Geometry: final body of the model. Coordinates: model frame, mm. Face numbers are marked on the shaded views. A direction names the side the tool comes from. Coordinates: 2 decimals unless noted, no trailing zeros. Order: outer loops, then holes, each group sorted by start corner. A loop starts at its lowest first (then second) coordinate and runs counter-clockwise, first axis right, second up. Notation, with made-up numbers: (-30, 38.25) - (-16, 38.25) arc R24 ccw to (-16, 68.25) - close; hole circle Ø9 at (5, -36.5). An arc over 180 degrees is marked (long way). Use a Markdown table: item, result. Add a question column.
```python
from build123d import *

# Parameters (mm, degrees)
REVOLUCI_N1_ANGLE           = 180
SALIENTE_EXTRUIR1_DEPTH     = 15
CROQUIS4_R                  = 4
CORTAR_EXTRUIR1_DEPTH       = 139.387389496
REVOLUCI_N2_ANGLE           = 10
REVOLUCI_N2_OTHER_WAY_ANGLE = 10
CORTAR_EXTRUIR2_DEPTH       = 10
CROQUIS7_R                  = 2
CORTAR_EXTRUIR3_DEPTH       = 125.891504895
CORTAR_EXTRUIR4_DEPTH       = 141.925841064
REDONDEO1_R                 = 4


with BuildPart() as part:
    # Croquis1 → Revolución1 (revolve)
    with BuildSketch(Plane(origin=(0, 0, 0), x_dir=(0, 0, -1), z_dir=(1, 0, 0))):
        with BuildLine():
            Line((-25.795554958, 35.816642159), (-40.313941934, 90))
            Line((-40.313941934, 90), (-34.102284852, 90))
            Line((-34.102284852, 90), (-20, 37.36955643))
            ThreePointArc((-20, 37.36955643), (-12.468451731, 20.723921943), (0, 7.36955643))
            Line((0, 7.36955643), (0, 0))
            ThreePointArc((0, 0), (-16.178409273, 15.545572574), (-25.795554958, 35.816642159))
        make_face()
    revolve(axis=Axis((0, 7.36955643, 0), (0, -1, 0)), revolution_arc=REVOLUCI_N1_ANGLE)

    # Croquis3 → Saliente-Extruir1 (add)
    with BuildSketch(Plane(origin=(0, 90, 0), x_dir=(1, 0, 0), z_dir=(0, 1, 0))):
        with BuildLine():
            Line((-10, -32.603156782), (-10, -39.053987175))
            ThreePointArc((-10, -39.053987175), (-5.039530881, -39.997712969), (0, -40.313941934))
            Line((0, -40.313941934), (10, -40.313941934))
            Line((10, -40.313941934), (10, -34.102284852))
            Line((10, -34.102284852), (0, -34.102284852))
            ThreePointArc((0, -34.102284852), (-5.055872451, -33.72542047), (-10, -32.603156782))
        make_face()
        with BuildLine():
            Line((-10, 32.603156782), (-10, 39.053987175))
            ThreePointArc((-10, 39.053987175), (-5.039530881, 39.997712969), (0, 40.313941934))
            Line((0, 40.313941934), (10, 40.313941934))
            Line((10, 40.313941934), (10, 34.102284852))
            Line((10, 34.102284852), (0, 34.102284852))
            ThreePointArc((0, 34.102284852), (-5.055872451, 33.72542047), (-10, 32.603156782))
        make_face()
    extrude(amount=SALIENTE_EXTRUIR1_DEPTH)

    # Croquis4 → Cortar-Extruir1 (cut, through all)
    with BuildSketch(Plane.XY.offset(40.313941934)):
        with Locations(Location((0, 97.5, 0), (0, 0, 270))):
            Circle(CROQUIS4_R)
    extrude(amount=-CORTAR_EXTRUIR1_DEPTH, mode=Mode.SUBTRACT)

    # Croquis5 → Revolución2 (revolve)
    with BuildSketch(Plane.XY):
        Polygon((-40.313941934, 90), (-48.313941934, 90), (-45.63445001, 80), (-37.63445001, 80), align=None)
    revolve(axis=Axis((0, 0, 0), (0, 1, 0)), revolution_arc=REVOLUCI_N2_ANGLE)

    # Croquis5 → Revolución2 other way (revolve)
    with BuildSketch(Plane.XY):
        Polygon((-40.313941934, 90), (-48.313941934, 90), (-45.63445001, 80), (-37.63445001, 80), align=None)
    revolve(axis=Axis((0, 0, 0), (0, -1, 0)), revolution_arc=REVOLUCI_N2_OTHER_WAY_ANGLE)

    # Croquis6 → Cortar-Extruir2 (cut)
    with BuildSketch(Plane(origin=(0, 90, 0), x_dir=(1, 0, 0), z_dir=(0, 1, 0))):
        Polygon((-39.701482571, 7.000442551), (-47.80408758, 7.000442551), (-47.579944596, 8.389627973), align=None)
        Polygon((-39.701482571, -7.000442551), (-47.80408758, -7.000442551), (-47.579944596, -8.389627973), align=None)
    extrude(amount=-CORTAR_EXTRUIR2_DEPTH, mode=Mode.SUBTRACT)


with BuildPart() as cortar_extruir2_kept_piece:
    # of the separate pieces the step leaves, the one the design keeps (cortar_extruir2_pieces_kept)
    add(part.part.solids().sort_by_distance((0, 0, 0))[0])

    # Croquis7 → Cortar-Extruir3 (cut, through all)
    with BuildSketch(Plane.XY.offset(7.000442551)):
        with Locations((-42.701482571, 85)):
            Circle(CROQUIS7_R)
    extrude(amount=-CORTAR_EXTRUIR3_DEPTH, mode=Mode.SUBTRACT)

    # Croquis8 → Cortar-Extruir4 (cut, through all)
    with BuildSketch(Plane.XY.offset(40.313941934)):
        with BuildLine():
            Line((7.5, 97.5), (7.5, 105))
            Line((7.5, 105), (10, 105))
            Line((10, 105), (10, 90))
            Line((10, 90), (0, 90))
            ThreePointArc((0, 90), (5.303300859, 92.196699141), (7.5, 97.5))
        make_face()
    extrude(amount=-CORTAR_EXTRUIR4_DEPTH, mode=Mode.SUBTRACT)

    # Redondeo1
    redondeo1_edges = [cortar_extruir2_kept_piece.edges().sort_by_distance(p)[0] for p in [
        (7.5, 105, -37.208113393),
        (7.5, 105, 37.208113393),
        (-10, 105, -35.828571978),
        (-10, 105, 35.828571978),
        (-45.63445001, 80, 0),
        (-48.313941934, 90, 0),
    ]]
    fillet(redondeo1_edges, radius=REDONDEO1_R)


solid = cortar_extruir2_kept_piece.part
```
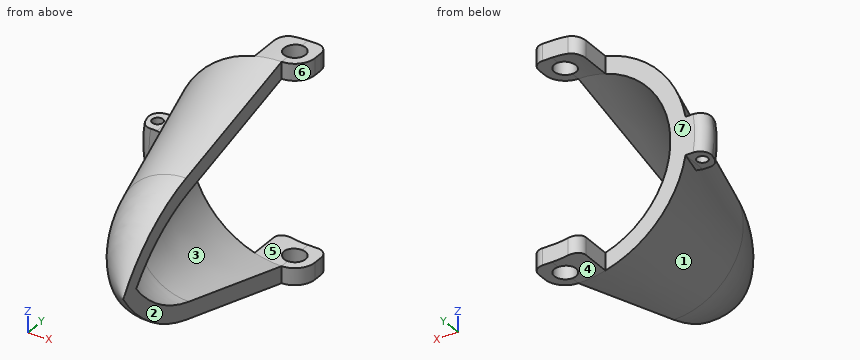
1) Section query A-A (y = 46.5). Return the cut outline in (x, z), and give its area (3 significant figures).
2) Access query for the marked faces 5, 6 and 7. Directions: +Z, -Z, +X, -X, +Y, -Y. A direction counts if a zero-diameter tool reaches every point of the face in a straight line with its end or side. Return the directions, or none.
3) Line query: line 1 (Z direction, x = 5.5, y = 93); line 2 (X direction, y = 97.5, z = -39); line 3 (Z direction, x = -1, y = 77.5). Output: solid intervals per line, ascending. Write a range as from..to.
4) First-contact query: pin 1 (8 mm diameter, centred on y = 35.5, z = 17, fed in from -X); pin 2 (6 mm diameter, centred on x = -41, z = 0.5, fed in from -Y); pin 3 (6 mm diameter, centred on y = 19, z = -23.5, fed in from -X); pin 4 (3 mm diameter, centred on y = 67, z = -1.5, fed in from -X) (3 decimals). Flat tips, straight axial feed; report the tip coordinate or a pass-through.
5) Draft query along Z for the marked faces 1, 2, 3 and 4. Return one class per face: released by +Z, released by -Z, zero draft, split by the parting line, or undercut.
From the geometry:
| question | item | result |
|---|---|---|
| 1 | outline | (0, -28.66) - (0, -22.45) arc R22.45 cw to (0, 22.45) - (0, 28.66) arc R28.66 ccw to start |
| 1 | area | 499 mm^2 |
| 2 | face 5 | +X, +Y |
| 2 | face 6 | +Z, -Z, +X, -Y |
| 2 | face 7 | +Z, -Z, -X, +Y |
| 3 | line 1 | z = -40.31..-34.1, 34.1..40.31 |
| 3 | line 2 | x = -10..-4, 4..7.5 |
| 3 | line 3 | z = -36.95..-30.74, 30.74..36.95 |
| 4 | pin 1 | stops at x = -22.49 |
| 4 | pin 2 | stops at y = 80 |
| 4 | pin 3 | passes through |
| 4 | pin 4 | stops at x = -34.525 |
| 5 | face 1 | split by the parting line |
| 5 | face 2 | zero draft |
| 5 | face 3 | undercut |
| 5 | face 4 | released by -Z |
